Build history of the part. All positions in model axes, mm. A direction names the side the tool comes from. Give positions to 0.01 mm unless a question says otherwise; leave off trailing zeros. Loops run counter-clockwise (first coordinate to the right, second up) from the corner with the lowest first, then second, coordinate; pieces in that order, holes last. Notation, with made-up numbers: (57, 10) -> (74, 10) arc R27 ccw to (74, 39) -> close; hole circle Ø1 at (-37, -31). An arc over 180 degrees is marked (long way). Answer as a JSON object with one key per item and string values. Group by question number.
Q1. Band-saw the part on D-D, the plane y = -13.5. Write the cut outline in (x, z), plus the area to 3 significant figures.
Q2. Band-saw the part on A-A, the plane z = 16.25. Write the cut outline in (x, y).
Q3. Two-plate mould, pull along X, no slides. Class faces 1 (the flat face through (-1, -75, 16)), 2 (the flat face through (-67.5, -1, 14)), 3 (the flat face through (-1, -80, 14)): pulls with the +X half, pulls with the -X half, needs draft (parallel to the pull), parting line crosses it, or undercut.
Q4. Band-saw the part on C-C, the plane x = -8.5. Write the cut outline in (y, z).
Q5. Drop flat-ended pins along their axis: pin 1 (6 mm diameter, centred on x = 16.5, y = 165.5, fed in from +Z); pin 2 (8 mm diameter, centred on y = 111.5, z = 3.5, fed in from -X); pin 3 (5 mm diameter, centred on x = -28, z = 4.5, fed in from +Y). Give the stop position or say it passes through.
Q6. Tool access for faces 4 (the flat face through (62.5, -1, 16)), 5 (the flat face through (14, 147, 5)), 6 (the flat face through (-18.5, 132.2, 2.5)), 7 (the cylindrical face through (0.482, 211.217, 2.465)): list every direction of +Z, -Z, +X, -X, +Y, -Y with a clear straight run to the whole face (end or side of a thin tool).
Q7. Band-saw the part on B-B, the plane y = 85. Write the cut outline in (x, z), plus the area to 3 significant figures.
Q8. Wall check: probe 1 along Y at (x, z) = (2, 22); probe 2 along X at (y, z) = (21, 17); probe 3 along Z at (x, y) = (17, 62). Give the ranges that are in metal, low to high. Write a range as from..to.
from build123d import *

# Parameters (mm, degrees)
BOSS_EXTRUDE1_DEPTH = 5
SKETCH2_W           = 135
SKETCH2_H           = 160
SKETCH2_W_2         = 125
SKETCH2_H_2         = 150
BOSS_EXTRUDE2_DEPTH = 23


with BuildPart() as part:
    # Sketch1 → Boss-Extrude1 (new body)
    with BuildSketch(Plane.XY):
        with BuildLine():
            Line((-67.5, 80), (-67.5, -80))
            Line((-67.5, -80), (67.5, -80))
            Line((67.5, -80), (67.5, 80))
            Line((67.5, 80), (26.490666647, 192.672217375))
            ThreePointArc((26.490666647, 192.672217375), (0, 211.221181853), (-26.490666647, 192.672217375))
            Line((-26.490666647, 192.672217375), (-67.5, 80))
        make_face()
        Polygon((-37.5, 80), (37.5, 80), (0, 183.03040323), align=None, mode=Mode.SUBTRACT)
    extrude(amount=BOSS_EXTRUDE1_DEPTH)

    # Sketch2 → Boss-Extrude2 (add)
    with BuildSketch(Plane.XY.offset(5)):
        Rectangle(SKETCH2_W, SKETCH2_H)
        Rectangle(SKETCH2_W_2, SKETCH2_H_2, mode=Mode.SUBTRACT)
    extrude(amount=BOSS_EXTRUDE2_DEPTH)


solid = part.part
Worked answers:
{
 "1": {"outline": "(-67.5, 0) -> (67.5, 0) -> (67.5, 28) -> (62.5, 28) -> (62.5, 5) -> (-62.5, 5) -> (-62.5, 28) -> (-67.5, 28) -> close", "area": "905 mm2"},
 "2": {"outline": "(-67.5, -80) -> (67.5, -80) -> (67.5, 80) -> (-67.5, 80) -> close; hole (-62.5, -75) -> (62.5, -75) -> (62.5, 75) -> (-62.5, 75) -> close"},
 "3": {"face 1": "undercut", "face 2": "pulls with the -X half", "face 3": "needs draft"},
 "4": {"outline": "(-80, 0) -> (80, 0) -> (80, 28) -> (75, 28) -> (75, 5) -> (-75, 5) -> (-75, 28) -> (-80, 28) -> close; (159.68, 0) -> (209.91, 0) -> (209.91, 5) -> (159.68, 5) -> close"},
 "5": {"pin 1": "z = 5", "pin 2": "x = -57.49", "pin 3": "y = 195.05"},
 "6": {"face 4": "+Z", "face 5": "+Z, +X, -X, +Y", "face 6": "+Z, -Z", "face 7": "+Z, -Z, +Y"},
 "7": {"outline": "(-65.68, 0) -> (-35.68, 0) -> (-35.68, 5) -> (-65.68, 5) -> close; (35.68, 0) -> (65.68, 0) -> (65.68, 5) -> (35.68, 5) -> close", "area": "300 mm2"},
 "8": {"probe 1": "-80..-75, 75..80", "probe 2": "-67.5..-62.5, 62.5..67.5", "probe 3": "0..5"}
}
